```python
from build123d import *

# Parameters (mm, degrees)
SKETCH1_W          = 168.4
SKETCH1_H          = 260
EXTRUDE1_DEPTH     = 4
SKETCH2_R          = 58.5
SKETCH2_R_2        = 2
CUT_EXTRUDE5_DEPTH = 4


with BuildPart() as part:
    # Sketch1 → Extrude1 (new body)
    with BuildSketch(Plane.XY):
        Rectangle(SKETCH1_W, SKETCH1_H)
    extrude(amount=EXTRUDE1_DEPTH)

    # Sketch2 → Cut-Extrude5 (cut)
    with BuildSketch(Plane.XY):
        Circle(SKETCH2_R)
        with Locations((-52.5, -52.5)):
            Circle(SKETCH2_R_2)
        with Locations((52.5, -52.5)):
            Circle(SKETCH2_R_2)
        with Locations((52.5, 52.5)):
            Circle(SKETCH2_R_2)
        with Locations((-52.5, 52.5)):
            Circle(SKETCH2_R_2)
    extrude(amount=CUT_EXTRUDE5_DEPTH, mode=Mode.SUBTRACT)


solid = part.part
```
The model under review builds one solid part; all positions refer to its coordinate system, in mm. Round coordinates to 2 decimals unless told otherwise and drop trailing zeros. Loops run counter-clockwise (first coordinate to the right, second up) from the corner with the lowest first, then second, coordinate; pieces in that order, holes last.
Item 1: Take a section at A-A (y = 0). Write out the cut boundary in (x, z).
Determined:
outline: (-84.2, 0) - (-58.5, 0) - (-58.5, 4) - (-84.2, 4) - close; (58.5, 0) - (84.2, 0) - (84.2, 4) - (58.5, 4) - close
Item 2: For line 1 (Y direction, x = 0, z = 0.95); line 2 (Y direction, x = 52.5, z = 1.8); line 3 (Y direction, x = -52, z = 1.9), list the stretches that pass through material, from the lowest coordinate up.
Determined:
line 1: y = -130 to -58.5, 58.5 to 130
line 2: y = -130 to -54.5, -50.5 to -25.81, 25.81 to 50.5, 54.5 to 130
line 3: y = -130 to -54.44, -50.56 to -26.8, 26.8 to 50.56, 54.44 to 130
Item 3: Clearance check with a flat-ended pin moving along its axis: pin 1 Ø3.5 at (x, y) = (52.5, -52.5) entering from +Z (3 decimals). State where the tip first meets the part, or that it passes through.
Determined:
pin 1: passes through
Item 4: Take a section at C-C (z = 2.6). Write out the cut boundary in (x, y).
Determined:
outline: (-84.2, -130) - (84.2, -130) - (84.2, 130) - (-84.2, 130) - close; hole circle Ø117 at (0, 0); hole circle Ø4 at (-52.5, -52.5); hole circle Ø4 at (-52.5, 52.5); hole circle Ø4 at (52.5, -52.5); hole circle Ø4 at (52.5, 52.5)
Item 5: Take a section at B-B (x = -4.5). Write out the cut boundary in (y, z), then the cut area to 3 significant figures.
Determined:
outline: (-130, 0) - (-58.33, 0) - (-58.33, 4) - (-130, 4) - close; (58.33, 0) - (130, 0) - (130, 4) - (58.33, 4) - close
area: 573 mm2
